The figure shows three views and two pictorial views of one solid part (mm, origin at its lowest corner). Answer the questions. A direction names the side the tool comes from. Coordinates: 2 decimals unless noted, no trailing zeros. Write each loop counter-clockwise with the first axis right and the second up, starting at its lowest first coordinate (ties: lowest second). Pieces come first, ordered by that corner, then holes. Notation, with made-up numbers: M -30,-4 L 13,-4 A27 cw 13,14 Z; hole C -35,-17.75 d7. An arc over 180 degrees is marked long. Use a Markdown table: item, result. Add a question column.
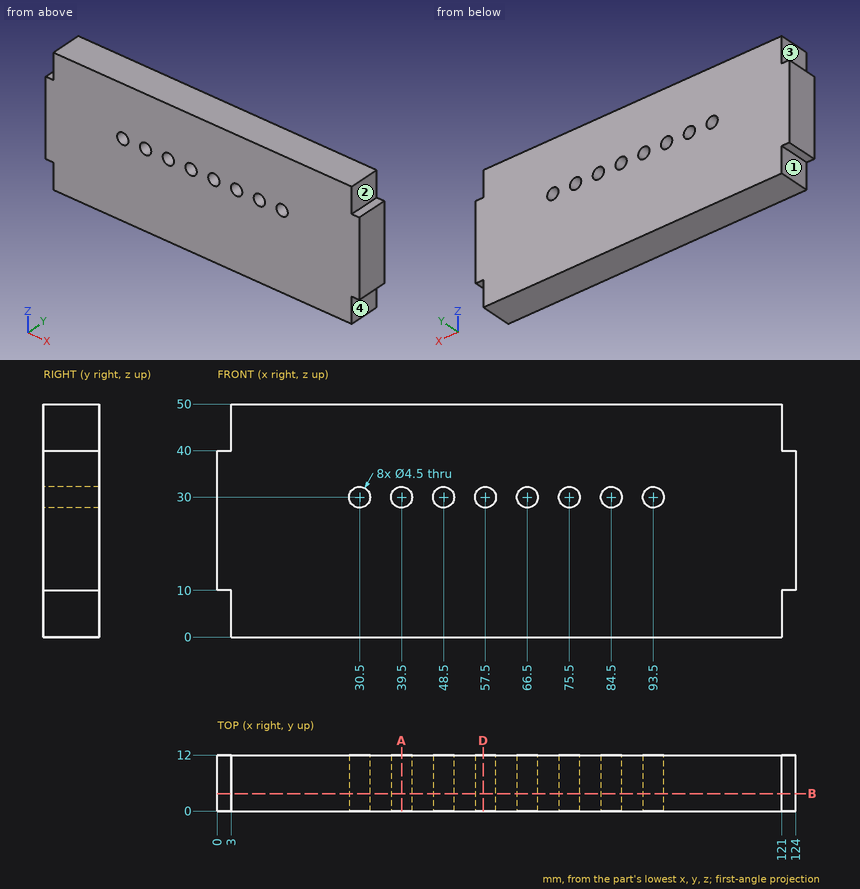
Item 1: Find section B-B on y = 3.75. Count the separate pieces of the cut face and the enclosed holes in it, then the cut area to 3 significant figures.
Item 2: Each of these flat-tipped pins is pushed along its axis until it touches: pin 1 (0.9 mm diameter, centred on x = 123, y = 4, fed in from -Z); pin 2 (6 mm diameter, centred on y = 2.5, z = 37.5, fed in from -X); pin 3 (1.5 mm diameter, centred on x = 1.5, y = 7, fed in from +Z); pin 4 (3 mm diameter, centred on y = 4.5, z = 3.5, fed in from +X). Where does it stop, or does it pass through?
Item 3: Find section A-A on x = 39.5. Give the vertices of the cut face in (y, z), then the cut area to 3 significant figures.
Item 4: Consider probe 1 along Z at (x, y) = (66.5, 8.5); probe 2 along X at (y, z) = (5, 6.5); probe 3 along Z at (x, y) = (47.5, 10.5). Determine where each line is inside the solid, lowest interval first.
Item 5: For the marked faces 1, 2, 3 and 4, determine the directions among +Z, -Z, +X, -X, +Y, -Y from which every point of the face is accessible in a straight line to the end or side of a thin tool.
Item 6: Find section D-D on x = 57. Give the vertices of the cut face in (y, z).
Geometry says:
| question | item | result |
|---|---|---|
| 1 | separate pieces | 1 |
| 1 | enclosed holes | 8 |
| 1 | area | 5,950 mm2 |
| 2 | pin 1 | stops at z = 10 |
| 2 | pin 2 | stops at x = 0 |
| 2 | pin 3 | stops at z = 40 |
| 2 | pin 4 | stops at x = 121 |
| 3 | outline | M 0,0 L 12,0 L 12,27.75 L 0,27.75 Z; M 0,32.25 L 12,32.25 L 12,50 L 0,50 Z |
| 3 | area | 546 mm2 |
| 4 | probe 1 | z = 0 to 27.75, 32.25 to 50 |
| 4 | probe 2 | x = 3 to 121 |
| 4 | probe 3 | z = 0 to 27.98, 32.02 to 50 |
| 5 | face 1 | -Z, -X, +Y, -Y |
| 5 | face 2 | +Z, +X, +Y, -Y |
| 5 | face 3 | +Z, -X, +Y, -Y |
| 5 | face 4 | -Z, +X, +Y, -Y |
| 6 | outline | M 0,0 L 12,0 L 12,27.81 L 0,27.81 Z; M 0,32.19 L 12,32.19 L 12,50 L 0,50 Z |
